```python
from build123d import *

# Parameters (mm, degrees)
LOW_START                          = 0.5
LOW_SCREW_HEAD_PROFILE_R           = 2.85
LOW_SCREW_HEAD_DEPTH               = 1.65
M3_START                           = -4.5
M3_SHANK_THREADS_OMITTED_PROFILE_R = 1.5
M3_SHANK_THREADS_OMITTED_DEPTH     = 5
M3_WASHER_ENVELOPE_PROFILE_R       = 3.5
M3_WASHER_ENVELOPE_PROFILE_R_2     = 1.7
M3_WASHER_ENVELOPE_DEPTH           = 0.5


with BuildPart() as part:
    # Low screw head profile → Low screw head (new body)
    with BuildSketch(Plane.XY.offset(LOW_START)):
        Circle(LOW_SCREW_HEAD_PROFILE_R)
    extrude(amount=LOW_SCREW_HEAD_DEPTH)

    # M3 shank, threads omitted profile → M3 shank, threads omitted (add)
    with BuildSketch(Plane.XY.offset(M3_START)):
        Circle(M3_SHANK_THREADS_OMITTED_PROFILE_R)
    extrude(amount=M3_SHANK_THREADS_OMITTED_DEPTH)

    # M3 washer envelope profile → M3 washer envelope (add)
    with BuildSketch(Plane.XY):
        Circle(M3_WASHER_ENVELOPE_PROFILE_R)
        Circle(M3_WASHER_ENVELOPE_PROFILE_R_2, mode=Mode.SUBTRACT)
    extrude(amount=M3_WASHER_ENVELOPE_DEPTH)


solid = part.part
```
Input: part model. Units: mm. Frame: model coordinates. A direction names the side the tool comes from. Round coordinates to 2 decimals unless told otherwise and drop trailing zeros. Write each loop counter-clockwise with the first axis right and the second up, starting at its lowest first coordinate (ties: lowest second). Pieces come first, ordered by that corner, then holes. Notation, with made-up numbers: M 15,-19 L 33,-19 A27 ccw 33,1 Z; hole C -10,73.5 d5. An arc over 180 degrees is marked long. Write each question's results on one line, items separated by ' | '.
Q1. Section query C-C (z = -3.5). Return loops of the section in (x, y).
Results:
outline: C 0,0 d3
Q2. Line query: line 1 along Y through (x, z) = (0, 0.3); line 2 along Z through (x, y) = (2, -1.25); line 3 along Y through (x, z) = (0, -3.75). Output: solid intervals per line, ascending.
Results:
line 1: y = -3.5 to -1.7, -1.5 to 1.5, 1.7 to 3.5 | line 2: z = 0 to 2.15 | line 3: y = -1.5 to 1.5
Q3. Draft query along X for faces 1 (the face through (3.233, -1.341, 0.246)), 2 (the face through (0, 0, 2.15)), 3 (the face through (-0.37, -1.66, 0.25)). Return one class per face: released by +X, released by -X, zero draft, split by the parting line, or undercut.
Results:
face 1: split by the parting line | face 2: zero draft | face 3: undercut
Q4. Section query D-D (y = -2.25). Return loops of the section in (x, z), and give its area (3 significant figures).
Results:
outline: M -2.68,0 L 2.68,0 L 2.68,0.5 L 1.75,0.5 L 1.75,2.15 L -1.75,2.15 L -1.75,0.5 L -2.68,0.5 Z | area: 8.45 mm^2
Q5. Access query for faces 4 (the face through (-1.5, 0.07, -2.04)), 5 (the face through (-1, -3, 0.5)), 6 (the face through (0, 0, -4.5)). Directions: +Z, -Z, +X, -X, +Y, -Y. A direction counts if a zero-diameter tool reaches every point of the face in a straight line with its end or side. Return the directions, or none.
Results:
face 4: -Z | face 5: +Z | face 6: -Z, +X, -X, +Y, -Y
Q6. Pin query (flat end, axial travel): P1, Ø2, axis at y = 0, z = -0.5, coming from the +X side; P2, Ø2, axis at x = 1, y = 2.5, coming from the -Z side; P3, Ø3, axis at y = 2.5, z = -3.5, coming from the -X side. Return the tip coordinate at first contact, or that it passes through.
Results:
P1: stops at x = 3.5 | P2: stops at z = 0 | P3: stops at x = -1.12
Q7. Section query A-A (y = 0). Return loops of the section in (x, z).
Results:
outline: M -3.5,0 L -1.7,0 L -1.7,0.5 L -1.5,0.5 L -1.5,-4.5 L 1.5,-4.5 L 1.5,0.5 L 1.7,0.5 L 1.7,0 L 3.5,0 L 3.5,0.5 L 2.85,0.5 L 2.85,2.15 L -2.85,2.15 L -2.85,0.5 L -3.5,0.5 Z
